Autodesk Inventor part; units mm, degrees
ref_plane "YZ Plane" through (0, 0, 0) normal (1, 0, 0) x (0, 1, 0)
ref_plane "XZ Plane" through (0, 0, 0) normal (0, 1, 0) x (-1, 0, 0)
ref_plane "XY Plane" through (0, 0, 0) normal (0, 0, 1) x (1, 0, 0)
sketch "Esboço1" plane through (0, 0, 0) normal (0, 0, 1) x (1, 0, 0)
  circle A0 centre (0, 0) radius 25
  circle A1 centre (0, 0) radius 8
  dimension "d0" = 50
  dimension "d1" = 16
extrude "Extrusão1" add sketch "Esboço1" along normal blind 5
sketch "Esboço2" plane through (0, 0, 5) normal (0, 0, 1) x (1, 0, 0)
  circle A0 centre (0, 0) radius 14 construction
  circle A1 centre (0, 0) radius 25 construction
  line L0 (0, 25) -> (0, 14) construction
  circle A2 centre (0, 19.5) radius 2.25
  dimension "d4" = 28
  dimension "d5" = 4.5
extrude "Extrusão2" cut sketch "Esboço2" against normal through all
pattern_circular "Padrão circular1" count 3 over 360 about axis through (0, 0, 0) along (0, 0, 1) of "Extrusão2"
properties part number "Retentor"
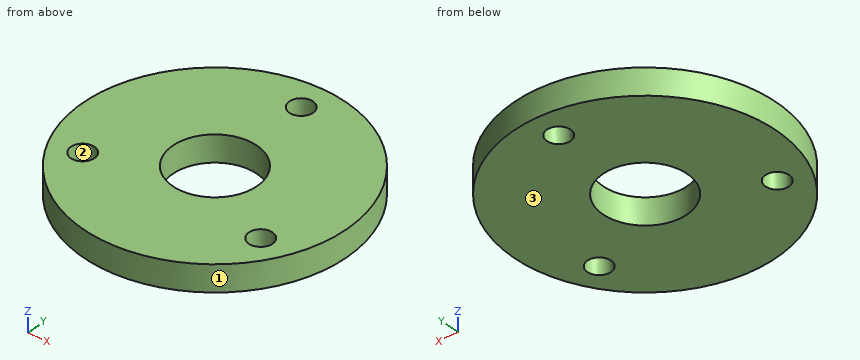
Geometry: final body of the model. Coordinates: model frame, mm. Face numbers are marked on the shaded views. Coordinates: 2 decimals unless noted, no trailing zeros. Loops run counter-clockwise (first coordinate to the right, second up) from the corner with the lowest first, then second, coordinate; pieces in that order, holes last. Notation, with made-up numbers: (-1, 1) -> (17, 1) arc R7 ccw to (17, 12) -> close; hole circle Ø3 at (89.5, 8). An arc over 180 degrees is marked (long way). Use a Markdown table: item, result. Add a question column.
(1) Section query C-C, the plane x = -5. Return loops of the section in (y, z) (3 decimals).
(2) Section query D-D, the plane y = -9.75. Return loops of the section in (x, z), plus the area to 3 significant figures.
(3) Section query A-A, the plane x = 0. Return loops of the section in (y, z), plus the area to 4 significant figures.
(4) Mould query, pull axis X, two halves, no side actions, for the marked faces 1, 2 and 3. Classes: pulls with the +X half, pulls with the -X half, needs draft (parallel to the pull), parting line crosses it, or undercut.
(5) Section query B-B, the plane y = 0. Return loops of the section in (x, z), plus the area to 3 significant figures.
(6) Line query: line 1 along Y through (x, z) = (0, 2); line 2 along Y through (x, z) = (4.5, 4.5); line 3 along Y through (x, z) = (-1, 1.4). Output: solid intervals per line, ascending.
(7) Pin query (flat end, axial travel): pin 1 Ø1.5 at (x, z) = (-18.5, 0.5) entering from -Y; pin 2 Ø2 at (x, z) = (4, 4.5) entering from -Y; pin 3 Ø1 at (y, z) = (-9, 4) entering from -X. Return the tip coordinate at first contact, or that it passes through.
Answer:
| question | item | result |
|---|---|---|
| 1 | outline | (-24.495, 0) -> (-6.245, 0) -> (-6.245, 5) -> (-24.495, 5) -> close; (6.245, 0) -> (24.495, 0) -> (24.495, 5) -> (6.245, 5) -> close |
| 2 | outline | (-23.02, 0) -> (-19.14, 0) -> (-19.14, 5) -> (-23.02, 5) -> close; (-14.64, 0) -> (14.64, 0) -> (14.64, 5) -> (-14.64, 5) -> close; (19.14, 0) -> (23.02, 0) -> (23.02, 5) -> (19.14, 5) -> close |
| 2 | area | 185 mm^2 |
| 3 | outline | (-25, 0) -> (-8, 0) -> (-8, 5) -> (-25, 5) -> close; (8, 0) -> (17.25, 0) -> (17.25, 5) -> (8, 5) -> close; (21.75, 0) -> (25, 0) -> (25, 5) -> (21.75, 5) -> close |
| 3 | area | 147.5 mm^2 |
| 4 | face 1 | parting line crosses it |
| 4 | face 2 | undercut |
| 4 | face 3 | needs draft |
| 5 | outline | (-25, 0) -> (-8, 0) -> (-8, 5) -> (-25, 5) -> close; (8, 0) -> (25, 0) -> (25, 5) -> (8, 5) -> close |
| 5 | area | 170 mm^2 |
| 6 | line 1 | y = -25 to -8, 8 to 17.25, 21.75 to 25 |
| 6 | line 2 | y = -24.59 to -6.61, 6.61 to 24.59 |
| 6 | line 3 | y = -24.98 to -7.94, 7.94 to 17.48, 21.52 to 24.98 |
| 7 | pin 1 | stops at y = -17.61 |
| 7 | pin 2 | stops at y = -24.82 |
| 7 | pin 3 | stops at x = -23.51 |
